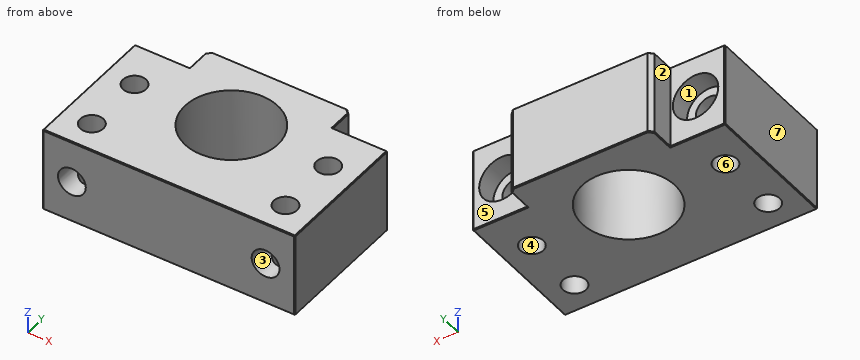
from build123d import *

# Parameters (mm, degrees)
SKETCH_1_W          = 60
SKETCH_1_H          = 32.5
EXTRUDE_1_DEPTH     = 20
SKETCH_2_W          = 34
SKETCH_2_H          = 20
EXTRUDE_2_DEPTH     = 6.5
SKETCH_3_R          = 5.4
CUT_EXTRUDE_1_DEPTH = 5
SKETCH_4_R          = 3.3
CUT_EXTRUDE_2_DEPTH = 46.345892868
SKETCH_7_R          = 2.75
CUT_EXTRUDE_3_DEPTH = 43.632880503
SKETCH_8_R          = 11
CUT_EXTRUDE_4_DEPTH = 35
CHAMFER_1_SIZE      = 1
CHAMFER_2_SIZE      = 0.2
CHAMFER_3_SIZE      = 0.2


with BuildPart() as part:
    # 草图1 → 凸台-拉伸1 (new body)
    with BuildSketch(Plane.XY):
        Rectangle(SKETCH_1_W, SKETCH_1_H)
    extrude(amount=EXTRUDE_1_DEPTH)

    # 草图2 → 凸台-拉伸2 (add)
    with BuildSketch(Plane(origin=(0, 16.25, 0), x_dir=(1, 0, 0), z_dir=(0, 1, 0))):
        with Locations((0, -10)):
            Rectangle(SKETCH_2_W, SKETCH_2_H)
    extrude(amount=EXTRUDE_2_DEPTH)

    # 草图3 → 切除-拉伸1 (cut)
    with BuildSketch(Plane(origin=(0, 16.25, 0), x_dir=(1, 0, 0), z_dir=(0, 1, 0))):
        with Locations(Location((-23, -10, 0), (0, 0, 270))):
            Circle(SKETCH_3_R)
        with Locations(Location((23, -10, 0), (0, 0, 270))):
            Circle(SKETCH_3_R)
    extrude(amount=-CUT_EXTRUDE_1_DEPTH, mode=Mode.SUBTRACT)

    # 草图4 → 切除-拉伸2 (cut, through all)
    with BuildSketch(Plane(origin=(0, 11.25, 0), x_dir=(1, 0, 0), z_dir=(0, 1, 0))):
        with Locations(Location((-23, -10, 0), (0, 0, 270))):
            Circle(SKETCH_4_R)
        with Locations(Location((23, -10, 0), (0, 0, 270))):
            Circle(SKETCH_4_R)
    extrude(amount=-CUT_EXTRUDE_2_DEPTH, mode=Mode.SUBTRACT)

    # 草图7 → 切除-拉伸3 (cut, through all)
    with BuildSketch(Plane.XY.offset(20)):
        with Locations((-23, 5.75)):
            Circle(SKETCH_7_R)
        with Locations((23, 5.75)):
            Circle(SKETCH_7_R)
        with Locations((-23, -9.25)):
            Circle(SKETCH_7_R)
        with Locations((23, -9.25)):
            Circle(SKETCH_7_R)
    extrude(amount=-CUT_EXTRUDE_3_DEPTH, mode=Mode.SUBTRACT)

    # 草图8 → 切除-拉伸4 (cut)
    with BuildSketch(Plane.XY.offset(20)):
        with Locations((0, 5.75)):
            Circle(SKETCH_8_R)
    extrude(amount=-CUT_EXTRUDE_4_DEPTH, mode=Mode.SUBTRACT)

    # 倒角1
    chamfer_1_edges = [part.edges().sort_by_distance(p)[0] for p in [
        (17, 22.75, 10),
        (-17, 22.75, 10),
    ]]
    chamfer(chamfer_1_edges, length=CHAMFER_1_SIZE)

    # 倒角2
    chamfer_2_edges = [part.edges().sort_by_distance(p)[0] for p in [
        (-16.5, 22.25, 0),
        (-17, 19, 0),
        (-23.5, 16.25, 0),
        (0, 22.75, 0),
        (16.5, 22.25, 0),
        (17, 19, 0),
        (23.5, 16.25, 0),
        (30, 16.25, 10),
        (23.5, 16.25, 20),
        (17, 19, 20),
        (16.5, 22.25, 20),
        (0, 22.75, 20),
        (-16.5, 22.25, 20),
        (-17, 19, 20),
        (-23.5, 16.25, 20),
        (-30, 16.25, 10),
    ]]
    chamfer(chamfer_2_edges, length=CHAMFER_2_SIZE)

    # 倒角3
    chamfer_3_edges = [part.edges().sort_by_distance(p)[0] for p in [
        (-30, -0.1, 0),
        (-30, -0.1, 20),
        (0, -16.25, 20),
        (30, -0.1, 20),
        (0, -16.25, 0),
        (30, -0.1, 0),
        (30, -16.25, 10),
        (-30, -16.25, 10),
    ]]
    chamfer(chamfer_3_edges, length=CHAMFER_3_SIZE)


solid = part.part
For this review, take the finished solid that the model builds, in its own axes (mm). Face numbers are marked on the shaded views. A direction names the side the tool comes from. Round coordinates to 2 decimals unless told otherwise and drop trailing zeros. Write each loop counter-clockwise with the first axis right and the second up, starting at its lowest first coordinate (ties: lowest second). Pieces come first, ordered by that corner, then holes. Notation, with made-up numbers: (67.25, -34.5) - (83.25, -34.5) arc R13 ccw to (83.25, -17.5) - close; hole circle Ø8 at (-1, 27). An arc over 180 degrees is marked (long way). Use a Markdown table: item, result.
Q1. Machinability: for the marked faces 1, 2 and 3, which of the approach directions +Z, -Z, +X, -X, +Y, -Y give a long, thin tool a straight path to every point of the face, cutting with its end or side? Answer none if there is none.
Derived:
| item | result |
|---|---|
| face 1 | +Y |
| face 2 | +Z, -Z, -X, +Y |
| face 3 | +Y, -Y |
Q2. Wall thickness on line 1 along X through (y, z) = (-9.25, 15.5); line 2 along X through (y, z) = (-7, 10); line 3 along Y through (x, z) = (-23, 15.5): over which ranges is each line inside the solid? List them lowest first.
Derived:
| item | result |
|---|---|
| line 1 | x = -30 to -25.75, -20.25 to 20.25, 25.75 to 30 |
| line 2 | x = -30 to -26.3, -19.7 to 19.7, 26.3 to 30 |
| line 3 | y = -16.25 to -12, -6.5 to 3, 8.5 to 16.25 |
Q3. We need section D-D (y = -9.25). Give the boundary of the cut face in (x, z).
Derived:
| item | result |
|---|---|
| outline | (-30, 0.2) - (-29.8, 0) - (-25.75, 0) - (-25.75, 8.18) arc R3.3 cw to (-25.75, 11.82) - (-25.75, 20) - (-29.8, 20) - (-30, 19.8) - close; (-20.25, 0) - (20.25, 0) - (20.25, 8.18) arc R3.3 cw to (20.25, 11.82) - (20.25, 20) - (-20.25, 20) - (-20.25, 11.82) arc R3.3 cw to (-20.25, 8.18) - close; (25.75, 0) - (29.8, 0) - (30, 0.2) - (30, 19.8) - (29.8, 20) - (25.75, 20) - (25.75, 11.82) arc R3.3 cw to (25.75, 8.18) - close |
Q4. We need section C-C (y = 5.75). Give the boundary of the cut face in (x, z).
Derived:
| item | result |
|---|---|
| outline | (-30, 0.2) - (-29.8, 0) - (-25.75, 0) - (-25.75, 8.18) arc R3.3 cw to (-25.75, 11.82) - (-25.75, 20) - (-29.8, 20) - (-30, 19.8) - close; (-20.25, 0) - (-11, 0) - (-11, 20) - (-20.25, 20) - (-20.25, 11.82) arc R3.3 cw to (-20.25, 8.18) - close; (11, 0) - (20.25, 0) - (20.25, 8.18) arc R3.3 cw to (20.25, 11.82) - (20.25, 20) - (11, 20) - close; (25.75, 0) - (29.8, 0) - (30, 0.2) - (30, 19.8) - (29.8, 20) - (25.75, 20) - (25.75, 11.82) arc R3.3 cw to (25.75, 8.18) - close |
Q5. The part is to be moulded in two halves that separate along Y. For the marked faces 4, 5, 6 and 7, say which applies: pulls with the +Y half, pulls with the -Y half, needs draft (parallel to the pull), parting line crosses it, or undercut.
Derived:
| item | result |
|---|---|
| face 4 | undercut |
| face 5 | pulls with the +Y half |
| face 6 | undercut |
| face 7 | needs draft |
Q6. Clearance check with flat-ended pins moving along their axes: pin 1 (10 mm diameter, centred on x = -20.5, z = 8.5, fed in from +Y); pin 2 (3.5 mm diameter, centred on x = -23, y = 5.75, fed in from -Z); pin 3 (6 mm diameter, centred on y = 20, z = 7.5, fed in from +X); pin 4 (6.5 mm diameter, centred on x = 24, z = 8.5, fed in from +Y). State where each tip first meets the part, or that it passes through.
Derived:
| item | result |
|---|---|
| pin 1 | stops at y = 22.75 |
| pin 2 | passes through |
| pin 3 | stops at x = 17 |
| pin 4 | stops at y = 11.25 |
Q7. We need section A-A (z = 10). State how many separate pieces and enclosed holes the cut face has, plus the area to 3 significant figures.
Derived:
| item | result |
|---|---|
| separate pieces | 3 |
| enclosed holes | 1 |
| area | 1,320 mm2 |
